Autodesk Inventor part; units mm, degrees
ref_plane "YZ Plane" through (0, 0, 0) normal (1, 0, 0) x (0, 1, 0)
ref_plane "XZ Plane" through (0, 0, 0) normal (0, 1, 0) x (-1, 0, 0)
ref_plane "XY Plane" through (0, 0, 0) normal (0, 0, 1) x (1, 0, 0)
sketch "Sketch1" plane through (0, 0, 0) normal (0, 0, 1) x (1, 0, 0)
  circle A0 centre (0, 0) radius 31.75
  dimension "d0" = 63.5
extrude "Extrusion1" add sketch "Sketch1" along normal blind 3.81
sketch "Sketch2" plane through (0, 0, 3.81) normal (0, 0, 1) x (1, 0, 0)
  line L0 (-11.1125, 19.2474) -> (11.1125, 19.2474)
  line L1 (11.1125, 19.2474) -> (22.225, 0)
  line L2 (22.225, 0) -> (11.1125, -19.2474)
  line L3 (11.1125, -19.2474) -> (-11.1125, -19.2474)
  line L4 (-11.1125, -19.2474) -> (-22.225, 0)
  line L5 (-22.225, 0) -> (-11.1125, 19.2474)
  line L6 (-12.5559, 21.7474) -> (-9.6691, 21.7474)
  line L7 (-9.6691, 21.7474) -> (-8.2257, 19.2474)
  line L8 (-8.2257, 19.2474) -> (-9.6691, 16.7474)
  line L9 (-9.6691, 16.7474) -> (-12.5559, 16.7474)
  line L10 (-12.5559, 16.7474) -> (-13.9993, 19.2474)
  line L11 (-13.9993, 19.2474) -> (-12.5559, 21.7474)
  line L12 (-23.6684, -2.5) -> (-25.1118, 0)
  line L13 (-25.1118, 0) -> (-23.6684, 2.5)
  line L14 (-23.6684, 2.5) -> (-20.7816, 2.5)
  line L15 (-20.7816, 2.5) -> (-19.3382, 0)
  line L16 (-19.3382, 0) -> (-20.7816, -2.5)
  line L17 (-20.7816, -2.5) -> (-23.6684, -2.5)
  line L18 (-9.6691, -21.7474) -> (-12.5559, -21.7474)
  line L19 (-12.5559, -21.7474) -> (-13.9993, -19.2474)
  line L20 (-13.9993, -19.2474) -> (-12.5559, -16.7474)
  line L21 (-12.5559, -16.7474) -> (-9.6691, -16.7474)
  line L22 (-9.6691, -16.7474) -> (-8.2257, -19.2474)
  line L23 (-8.2257, -19.2474) -> (-9.6691, -21.7474)
  line L24 (13.9993, -19.2474) -> (12.5559, -21.7474)
  line L25 (12.5559, -21.7474) -> (9.6691, -21.7474)
  line L26 (9.6691, -21.7474) -> (8.2257, -19.2474)
  line L27 (8.2257, -19.2474) -> (9.6691, -16.7474)
  line L28 (9.6691, -16.7474) -> (12.5559, -16.7474)
  line L29 (12.5559, -16.7474) -> (13.9993, -19.2474)
  line L30 (23.6684, 2.5) -> (25.1118, 0)
  line L31 (25.1118, 0) -> (23.6684, -2.5)
  line L32 (23.6684, -2.5) -> (20.7816, -2.5)
  line L33 (20.7816, -2.5) -> (19.3382, 0)
  line L34 (19.3382, 0) -> (20.7816, 2.5)
  line L35 (20.7816, 2.5) -> (23.6684, 2.5)
  line L36 (9.6691, 21.7474) -> (12.5559, 21.7474)
  line L37 (12.5559, 21.7474) -> (13.9993, 19.2474)
  line L38 (13.9993, 19.2474) -> (12.5559, 16.7474)
  line L39 (12.5559, 16.7474) -> (9.6691, 16.7474)
  line L40 (9.6691, 16.7474) -> (8.2257, 19.2474)
  line L41 (8.2257, 19.2474) -> (9.6691, 21.7474)
  point P0 (0, 0)
  point P1 (0, 0)
  point P2 (0, 0)
  dimension "d15" = 5
  dimension "d18" = 360
  dimension "d20" = 22.225
extrude "Extrusion2" cut sketch "Sketch2" against normal blind 3.81 contours L5 L10 L11 L6 L7 L0 | L0 L8 L9 L5 | L41 L36 L37 L38 L1 L0 | L0 L1 L39 L40 | L15 L16 L4 L5 | L5 L4 L17 L12 L13 L14 | L35 L30 L31 L32 L2 L1 | L1 L2 L33 L34 | L21 L22 L3 L4 | L4 L3 L23 L18 L19 L20 | L29 L24 L25 L26 L3 L2 | L2 L3 L27 L28
sketch "Sketch3" plane through (0, 0, 3.81) normal (0, 0, 1) x (1, 0, 0)
  circle A0 centre (0, 0) radius 31.75
  line L0 (-2.8868, 0) -> (-1.4434, 2.5)
  line L1 (-1.4434, 2.5) -> (1.4434, 2.5)
  line L2 (1.4434, 2.5) -> (2.8868, 0)
  line L3 (2.8868, 0) -> (1.4434, -2.5)
  line L4 (1.4434, -2.5) -> (-1.4434, -2.5)
  line L5 (-1.4434, -2.5) -> (-2.8868, 0)
  dimension "d14" = 5
extrude "Extrusion3" cut sketch "Sketch3" against normal blind 3.81 contours L0 L1 L2 L3 L4 L5
properties part number "Input _Ring"
Work out the finished part from the listing and answer in its coordinate system (mm). Give positions to 0.01 mm unless a question says otherwise; leave off trailing zeros. Write each loop counter-clockwise with the first axis right and the second up, starting at its lowest first coordinate (ties: lowest second). Pieces come first, ordered by that corner, then holes. Notation, with made-up numbers: (5, -26.75) - (40, -26.75) arc R21 ccw to (40, -7.75) - close; hole circle Ø3 at (-4.5, 47). An arc over 180 degrees is marked (long way). One line per item, written item: value. Start each with the question number.
1. Find section B-B (z = 1.2). State how many separate pieces and enclosed holes the cut face has, then the cut area to 3 significant figures.
2. Given pin 1 (1.4 mm diameter, centred on x = 11.5, z = 2.5, fed in from +Y); pin 2 (1.4 mm diameter, centred on x = 0.5, z = 2.5, fed in from +Y); pin 3 (1.4 mm diameter, centred on x = 21.5, z = 1, fed in from -Y), each flat-ended and moving along its own axis, determine where each tip first touches the part or whether it passes through.
3. Find section C-C (x = 22). Write down the section's boundary in (y, z).
4. Consider probe 1 along Y at (x, z) = (10.5, 3.05); probe 2 along Y at (x, z) = (11, 1); probe 3 along X at (y, z) = (-1, 1.75). Determine where each line is inside the solid, lowest interval first.
5. Find section A-A (x = 0). Write down the section's boundary in (y, z).
6. For a pull along Y with two mould halves and no side action, classify faces 1 (the cylindrical face through (-6.883, 30.995, 1.878)), 2 (the flat face through (22, -2.5, 2)) as +Y half, -Y half, draft (parallel to the pull), parting line (faces both ways), or undercut.
Geometry results:
1. separate pieces: 1
1. enclosed holes: 7
1. area: 3,020 mm2
2. pin 1: y = 29.86
2. pin 2: y = 31.75
2. pin 3: y = -23.99
3. outline: (-22.89, 0) - (-2.5, 0) - (-2.5, 3.81) - (-22.89, 3.81) - close; (2.5, 0) - (22.89, 0) - (22.89, 3.81) - (2.5, 3.81) - close
4. probe 1: -29.96 to -21.75, -16.75 to 16.75, 21.75 to 29.96
4. probe 2: -29.78 to -21.75, -16.75 to 16.75, 21.75 to 29.78
4. probe 3: -31.73 to -24.53, -19.92 to -2.31, 2.31 to 19.92, 24.53 to 31.73
5. outline: (-31.75, 0) - (-2.5, 0) - (-2.5, 3.81) - (-31.75, 3.81) - close; (2.5, 0) - (31.75, 0) - (31.75, 3.81) - (2.5, 3.81) - close
6. face 1: parting line
6. face 2: undercut
